The model under review builds one solid part; all positions refer to its coordinate system, in mm. Face numbers are marked on the shaded views. A direction names the side the tool comes from. Round coordinates to 2 decimals unless told otherwise and drop trailing zeros. Write each loop counter-clockwise with the first axis right and the second up, starting at its lowest first coordinate (ties: lowest second). Pieces come first, ordered by that corner, then holes. Notation, with made-up numbers: M 28,-18.5 L 35,-18.5 A28 cw 35,-0.5 Z; hole C 24.5,61 d4. An arc over 180 degrees is marked long. One line per item, written item: value. Start each with the question number.
1) Take a section at C-C, the plane z = 28.5. Write out the cut boundary in (x, y).
2) Take a section at A-A, the plane x = -15. Write out the cut boundary in (y, z), and give its area (3 significant figures).
3) For P1, Ø4, axis at x = 15, y = -6.5, coming from the -Z side; P2, Ø4, axis at y = -3.5, z = 26.5, coming from the -X side; P3, Ø3, axis at x = -15, y = -10, coming from the +Z side; P4, Ø6, axis at y = -8.5, z = 19, coming from the +X side, all flat-tipped, find the tip position at first contact; note any pin that passes through.
4) Tool access review of the marked faces 1, 2 and 3: name each direction out of +Z, -Z, +X, -X, +Y, -Y from which nothing blocks a thin tool from reaching the whole face with its end or side.
5) Take a section at B-B, the plane y = -10. State how many separate pieces and enclosed holes the cut face has, and give its area (3 significant figures).
6) Wall thickness on probe 1 along X at (y, z) = (-10, 1.05); probe 2 along X at (y, z) = (-1.25, 29.5); probe 3 along Y at (x, z) = (-15, 3): over which ranges is each line inside the solid? List them lowest first.
7) Take a section at D-D, the plane x = 3. Write out the cut boundary in (y, z).
from build123d import *

# Parameters (mm, degrees)
F1_DEPTH = 20
F2_R     = 2
F3_DEPTH = 25
F5_DEPTH = 8
F6_R     = 1.8
F7_DEPTH = 25
F8_R     = 2


with BuildPart() as f1:
    # F0 (on Front) → F1 (new body)
    with BuildSketch(Plane.XZ):
        with BuildLine():
            Line((-1, 33), (-10, 33))
            Line((-10, 33), (-10, 5))
            Line((-10, 5), (-20, 5))
            Line((-20, 5), (-20, 0))
            Line((-20, 0), (20, 0))
            Line((20, 0), (20, 5))
            Line((20, 5), (10, 5))
            Line((10, 5), (10, 33))
            Line((10, 33), (1, 33))
            Line((1, 33), (1, 24.3874821937))
            ThreePointArc((1, 24.3874821937), (3.5178118199, 22.8062430401), (4.5, 20))
            ThreePointArc((4.5, 20), (-2.8062430401, 16.4821881801), (-1, 24.3874821937))
            Line((-1, 24.3874821937), (-1, 33))
        make_face()
    extrude(amount=F1_DEPTH)

    # F2 (on face) → F3 (cut)
    with BuildSketch(Plane.YZ.offset(10)):
        with Locations((-10, 28.5)):
            Circle(F2_R)
    extrude(amount=-F3_DEPTH, mode=Mode.SUBTRACT)

    # F4 (on face) → F5 (cut)
    with BuildSketch(Plane.XY.offset(33)):
        Polygon((-7, -6.8), (-10, -6.8), (-10, -13.2), (-7, -13.2), (-7, -10), align=None)
    extrude(amount=-F5_DEPTH, mode=Mode.SUBTRACT)

    # F6 (on face) → F7 (cut)
    with BuildSketch(Plane(origin=(0, 0, 0), x_dir=(1, 0, 0), z_dir=(0, 0, -1))):
        with Locations((-15, 10)):
            Circle(F6_R)
        with Locations((15, 10)):
            Circle(F6_R)
    extrude(amount=-F7_DEPTH, mode=Mode.SUBTRACT)

    # F8
    f8_edges = [f1.edges().sort_by_distance(p)[0] for p in [
        (-10, -10, 5),
        (10, -10, 5),
        (-10, -16.6, 33),
        (10, -10, 33),
        (-10, -3.4, 33),
    ]]
    fillet(f8_edges, radius=F8_R)


solid = f1.part
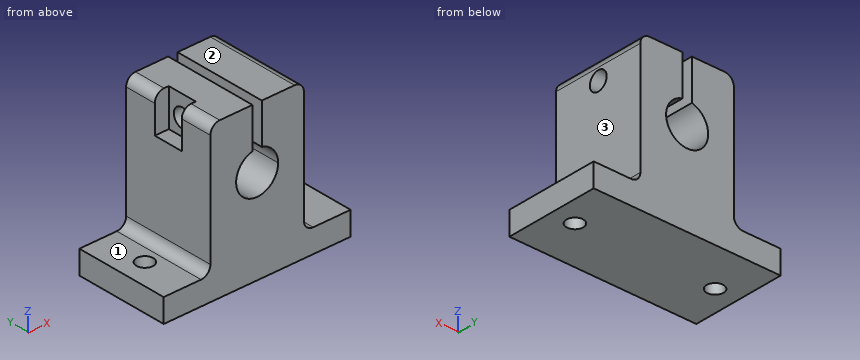
Checked values:
1. outline: M -10,-20 L -1,-20 L -1,-12 L -7,-12 L -7,-13.2 L -10,-13.2 Z; M -10,-6.8 L -7,-6.8 L -7,-8 L -1,-8 L -1,0 L -10,0 Z; M 1,-20 L 10,-20 L 10,-12 L 1,-12 Z; M 1,-8 L 10,-8 L 10,0 L 1,0 Z
2. outline: M -20,0 L -11.8,0 L -11.8,5 L -20,5 Z; M -8.2,0 L 0,0 L 0,5 L -8.2,5 Z
2. area: 82.0 mm2
3. P1: stops at z = 0
3. P2: stops at x = -10
3. P3: passes through
3. P4: stops at x = 10
4. face 1: +Z, -X, +Y, -Y
4. face 2: +Z, +X, -X, +Y, -Y
4. face 3: +Z, +X, +Y, -Y
5. separate pieces: 5
5. enclosed holes: 0
5. area: 560 mm2
6. probe 1: x = -20 to -16.8, -13.2 to 13.2, 16.8 to 20
6. probe 2: x = -10 to -1, 1 to 10
6. probe 3: y = -20 to -11.8, -8.2 to 0
7. outline: M -20,0 L 0,0 L 0,16.65 L -20,16.65 Z; M -20,23.35 L 0,23.35 L 0,33 L -20,33 Z; hole C -10,28.5 d4
